```python
from build123d import *

# Parameters (mm, degrees)
F0_W     = 60
F0_H     = 60
F1_DEPTH = 50
F2_W     = 40
F2_H     = 40
F3_DEPTH = 40
F4_W     = 50
F4_H     = 50
F5_DEPTH = 5


# Not quite as in the source:
# - a feature names something its author has since deleted; it is built from what else it names


with BuildPart() as f1:
    # F0 (on Top) → F1 (new body)
    with BuildSketch(Plane.XY):
        with Locations((30, 30)):
            Rectangle(F0_W, F0_H)
    extrude(amount=-F1_DEPTH)

    # F2 (on Top) → F3 (cut)
    with BuildSketch(Plane.XY):
        with Locations((30, 30)):
            Rectangle(F2_W, F2_H)
    extrude(amount=-F3_DEPTH, mode=Mode.SUBTRACT)

    # F4 (on Top) → F5 (cut)
    with BuildSketch(Plane.XY):
        with Locations((30, 30)):
            Rectangle(F4_W, F4_H)
    extrude(amount=-F5_DEPTH, mode=Mode.SUBTRACT)


solid = f1.part
```
Verification items for the finished model (mm, model axes). A direction names the side the tool comes from. Round coordinates to 2 decimals unless told otherwise and drop trailing zeros. Write each loop counter-clockwise with the first axis right and the second up, starting at its lowest first coordinate (ties: lowest second). Pieces come first, ordered by that corner, then holes. Notation, with made-up numbers: (56, -7) - (103, -7) arc R7 ccw to (103, -1) - close; hole circle Ø11 at (61.5, 37). An arc over 180 degrees is marked (long way). Answer as a JSON object with one key per item and string values. Group by question number.
Q1. Section check C-C, the plane z = -26.5. Enter the section's corners in (x, y).
Q2. Section check A-A, the plane x = 31. Enter the section's corners in (y, z).
Q3. Tool access check on faces 5 (the flat face through (30, 10, -22)), 6 (the flat face through (56, 30, 0)). Record the directions out of +Z, -Z, +X, -X, +Y, -Y that give a thin tool (end or side, any length) a straight path to the whole face; none if there is none.
Q4. Mould release check, pull along X, two halves, no side actions. Record for faces 1 (the flat face through (52, 30, -5)), 2 (the flat face through (55, 30, -2)), 3 (the flat face through (30, 30, -50)), 4 (the flat face through (60, 30, -25)): released by +X, released by -X, zero draft, split by the parting line, or undercut.
Q5. Section check B-B, the plane y = 7.5. Enter the section's corners in (x, z), plus the area to 3 significant figures.
Q6. Thickness scan on line 1 (X direction, y = 45, z = -23); line 2 (X direction, y = 40, z = -3). Record the ranges inside material, lowest first.
Q7. Go/stop test with a flat-tipped pin: pin 1 Ø20 at (x, y) = (29.5, 31.5) entering from +Z. Record where the tip stops, or that it passes through.
Found:
{
 "1": {"outline": "(0, 0) - (60, 0) - (60, 60) - (0, 60) - close; hole (10, 10) - (50, 10) - (50, 50) - (10, 50) - close"},
 "2": {"outline": "(0, -50) - (60, -50) - (60, 0) - (55, 0) - (55, -5) - (50, -5) - (50, -40) - (10, -40) - (10, -5) - (5, -5) - (5, 0) - (0, 0) - close"},
 "3": {"face 5": "+Z", "face 6": "+Z, +X, -X, +Y, -Y"},
 "4": {"face 1": "undercut", "face 2": "undercut", "face 3": "zero draft", "face 4": "released by +X"},
 "5": {"outline": "(0, -50) - (60, -50) - (60, 0) - (55, 0) - (55, -5) - (5, -5) - (5, 0) - (0, 0) - close", "area": "2,750 mm^2"},
 "6": {"line 1": "x = 0 to 10, 50 to 60", "line 2": "x = 0 to 5, 55 to 60"},
 "7": {"pin 1": "stops at z = -40"}
}
